CAD build for the part. Positions are in the model's coordinates, mm. A direction names the side the tool comes from. Give positions to 0.01 mm unless a question says otherwise; leave off trailing zeros. Order: outer loops, then holes, each group sorted by start corner. A loop starts at its lowest first (then second) coordinate and runs counter-clockwise, first axis right, second up.
```python
from build123d import *

# Parameters (mm, degrees)
F0_R     = 50
F1_DEPTH = 8
F2_R     = 26.25
F2_R_2   = 17.25
F3_DEPTH = 1.5
F4_R     = 5
F5_DEPTH = 15


with BuildPart() as f1:
    # F0 (on Top) → F1 (new body)
    with BuildSketch(Plane.XY):
        Circle(F0_R)
    extrude(amount=F1_DEPTH)

    # F2 (on face) → F3 (cut)
    with BuildSketch(Plane.XY.offset(8)):
        Circle(F2_R)
        Circle(F2_R_2, mode=Mode.SUBTRACT)
    extrude(amount=-F3_DEPTH, mode=Mode.SUBTRACT)

    # F4 (on face) → F5 (join)
    with BuildSketch(Plane.XY.offset(8)):
        Circle(F4_R)
    extrude(amount=F5_DEPTH)


solid = f1.part
```
Item 1: Slice it at A-A (y = 0). Give the cut face in (x, z), and give its area (3 significant figures).
Item 2: Slice it at D-D (x = -11.5). Give the cut face in (y, z).
Item 3: Drop flat-ended pins along their axis: pin 1 Ø5 at (y, z) = (31, 6) entering from +X; pin 2 Ø5 at (x, z) = (36.5, 5.5) entering from +Y; pin 3 Ø5 at (y, z) = (16.5, 9.5) entering from +X. Give the stop position or say it passes through.
Item 4: Tool access for faces 1 (the face through (0, 0, 23)), 2 (the face through (4, -4, 8)): list every direction of +Z, -Z, +X, -X, +Y, -Y with a clear straight run to the whole face (end or side of a thin tool).
Item 5: Wall check: L1, parallel to Y at x = 0, z = 7.4; L2, parallel to Z at x = 12.5, y = -14.5; L3, parallel to Z at x = -7.5, y = -33. Give the ranges that are in metal, low to high.
Item 6: Two-plate mould, pull along X, no slides. Class faces 3 (the face through (-1.08, -4.88, 15.4)), 4 (the face through (-1, 1, 0)), 5 (the face through (16.453, 5.181, 7.26)): released by +X, released by -X, zero draft, split by the parting line, or undercut.
Item 7: Slice it at C-C (z = 3.5). Give the cut face in (x, y).
A:
1. outline: (-50, 0) - (50, 0) - (50, 8) - (26.25, 8) - (26.25, 6.5) - (17.25, 6.5) - (17.25, 8) - (5, 8) - (5, 23) - (-5, 23) - (-5, 8) - (-17.25, 8) - (-17.25, 6.5) - (-26.25, 6.5) - (-26.25, 8) - (-50, 8) - close
1. area: 923 mm2
2. outline: (-48.66, 0) - (48.66, 0) - (48.66, 8) - (23.6, 8) - (23.6, 6.5) - (12.86, 6.5) - (12.86, 8) - (-12.86, 8) - (-12.86, 6.5) - (-23.6, 6.5) - (-23.6, 8) - (-48.66, 8) - close
3. pin 1: stops at x = 41.08
3. pin 2: stops at y = 36.66
3. pin 3: stops at x = 47.85
4. face 1: +Z, +X, -X, +Y, -Y
4. face 2: +Z
5. L1: y = -50 to -26.25, -17.25 to 17.25, 26.25 to 50
5. L2: z = 0 to 6.5
5. L3: z = 0 to 8
6. face 3: split by the parting line
6. face 4: zero draft
6. face 5: undercut
7. outline: circle Ø100 at (0, 0)
